Part model, mm, in its own coordinate system. A direction names the side the tool comes from. Coordinates: 2 decimals unless noted, no trailing zeros. Write each loop counter-clockwise with the first axis right and the second up, starting at its lowest first coordinate (ties: lowest second). Pieces come first, ordered by that corner, then holes. Notation, with made-up numbers: (-31.5, 42.5) -> (-22.5, 42.5) arc R18 ccw to (-22.5, 50.5) -> close; hole circle Ø10 at (75.25, 81). An arc over 180 degrees is marked (long way). Write item = value, one per line. Start each with the question number.
Q1. Pin check, flat tip, straight feed: P1, Ø1.5, axis at y = 365.5, z = -5, coming from the +X side. Stop position of the tip, or through.
Q2. Band-saw the part on B-B, the plane x = -12.7. Give the number of separate pieces and of enclosed holes in the cut face, plus the area to 3 significant figures.
Q3. Band-saw the part on C-C, the plane y = 209.55. List the corners of the cut face in (x, z).
Q4. Pull direction Z, two halves, no side cores. Call faces 3 (the cylindrical face through (-8.02, 16.99, -24.62)), 4 (the flat face through (-13, 219, 0)), 5 (the flat face through (-13, 219, -23.812)): released by +Z, released by -Z, zero draft, split by the parting line, or undercut.
Q5. Probe line 1 (Y direction, x = -12.7, z = -24.7); line 2 (X direction, y = 431.8, z = -24.35); line 3 (Z direction, x = -18.5, y = 244). List the from-to ranges inside material, lowest first.
Q6. Band-saw the part on A-A, the plane y = 12.7. List the corners of the cut face in (x, z).
Q7. Tool access for faces 1 (the flat face through (0, 219, -4)), 2 (the flat face through (-1.588, 219, -3)): list every direction of +Z, -Z, +X, -X, +Y, -Y with a clear straight run to the whole face (end or side of a thin tool).
Q8. Band-saw the part on D-D, the plane y = 105. List the corners of the cut face in (x, z), plus the area to 3 significant figures.
Autodesk Inventor part; units mm, degrees
ref_plane "YZ Plane" through (0, 0, 0) normal (1, 0, 0) x (0, 1, 0)
ref_plane "XZ Plane" through (0, 0, 0) normal (0, 1, 0) x (-1, 0, 0)
ref_plane "XY Plane" through (0, 0, 0) normal (0, 0, 1) x (1, 0, 0)
sketch "Sketch1" plane through (0, 0, 0) normal (0, 1, 0) x (-1, 0, 0)
  line L0 (0, 0) -> (25.4, 0)
  line L1 (25.4, 0) -> (25.4, -25.4)
  line L2 (25.4, -25.4) -> (0, -25.4)
  line L3 (0, -25.4) -> (0, 0)
  line L4 (23.8125, -23.8125) -> (23.8125, -1.5875)
  line L5 (23.8125, -1.5875) -> (1.5875, -1.5875)
  line L6 (1.5875, -1.5875) -> (1.5875, -23.8125)
  line L7 (1.5875, -23.8125) -> (23.8125, -23.8125)
  dimension "d0" = 25.4
  dimension "d1" = 25.4
  dimension "d2" = 1.5875
extrude "Extrusion1" add sketch "Sketch1" along normal blind 444.5
sketch "Sketch2" plane through (-25.4, 0, 0) normal (0, 0, 1) x (1, 0, 0)
  circle A0 centre (12.7, 431.8) radius 6.35
  line L0 (0, 444.5) -> (25.4, 444.5)
  point P0 (25.4, 0)
  dimension "d5" = 12.7
  dimension "d6" = 12.7
extrude "Extrusion2" cut sketch "Sketch2" against normal blind 25.4
sketch "Sketch4" plane through (0, 0, -25.4) normal (0, 0, -1) x (-1, 0, 0)
  circle A0 centre (12.7, 12.7) radius 6.35
  line L0 (25.4, 0) -> (0, 0)
  line L1 (0, 0) -> (0, 444.5)
  dimension "d17" = 12.7
  dimension "d18" = 12.7
  dimension "d19" = 12.7
extrude "Extrusion4" cut sketch "Sketch4" against normal blind 25.4
sketch "Sketch5" plane through (0, 0, -25.4) normal (0, 0, -1) x (-1, 0, 0)
  circle A0 centre (12.7, 209.55) radius 6.35
  line L0 (0, 0) -> (0, 444.5)
  line L1 (0, 444.5) -> (25.4, 444.5)
  dimension "d22" = 12.7
  dimension "d23" = 12.7
  dimension "d24" = 234.95
extrude "Extrusion5" cut sketch "Sketch5" against normal blind 25.4
sketch "Sketch6" plane through (0, 0, 0) normal (1, 0, 0) x (0, 0, -1)
  line L0 (5.08, 265.303) -> (20.32, 265.303)
  line L1 (20.32, 265.303) -> (20.32, 88.9)
  line L2 (20.32, 88.9) -> (5.08, 88.9)
  line L3 (5.08, 88.9) -> (5.08, 265.303)
  line L4 (23.8125, 444.5) -> (1.5875, 444.5)
  line L5 (25.4, 0) -> (25.4, 444.5)
  line L6 (0, 0) -> (0, 444.5)
  line L7 (25.4, 0) -> (0, 0)
  dimension "d28" = 5.08
  dimension "d29" = 5.08
  dimension "d30" = 176.403
  dimension "d33" = 88.9
extrude "Extrusion6" cut sketch "Sketch6" against normal blind 25.4
properties part number "AP 5"
Ans:
q1.P1 = 0
q2.separate_pieces = 8
q2.enclosed_holes = 0
q2.area = 1,290 mm2
q3.outline = (-25.4, -25.4) -> (-19.05, -25.4) -> (-19.05, -23.81) -> (-23.81, -23.81) -> (-23.81, -20.32) -> (-25.4, -20.32) -> close; (-25.4, -5.08) -> (-23.81, -5.08) -> (-23.81, -1.59) -> (-19.05, -1.59) -> (-19.05, 0) -> (-25.4, 0) -> close; (-6.35, -25.4) -> (0, -25.4) -> (0, -20.32) -> (-1.59, -20.32) -> (-1.59, -23.81) -> (-6.35, -23.81) -> close; (-6.35, -1.59) -> (-1.59, -1.59) -> (-1.59, -5.08) -> (0, -5.08) -> (0, 0) -> (-6.35, 0) -> close
q4.face_3 = zero draft
q4.face_4 = released by +Z
q4.face_5 = undercut
q5.line_1 = 0 to 6.35, 19.05 to 203.2, 215.9 to 425.45, 438.15 to 444.5
q5.line_2 = -25.4 to -19.05, -6.35 to 0
q5.line_3 = -25.4 to -23.81, -1.59 to 0
q6.outline = (-25.4, -25.4) -> (-19.05, -25.4) -> (-19.05, -23.81) -> (-23.81, -23.81) -> (-23.81, -1.59) -> (-19.05, -1.59) -> (-19.05, 0) -> (-25.4, 0) -> close; (-6.35, -25.4) -> (0, -25.4) -> (0, 0) -> (-6.35, 0) -> (-6.35, -1.59) -> (-1.59, -1.59) -> (-1.59, -23.81) -> (-6.35, -23.81) -> close
q7.face_1 = +Z, -Z, +X, +Y, -Y
q7.face_2 = +Y, -Y
q8.outline = (-25.4, -25.4) -> (0, -25.4) -> (0, -20.32) -> (-1.59, -20.32) -> (-1.59, -23.81) -> (-23.81, -23.81) -> (-23.81, -20.32) -> (-25.4, -20.32) -> close; (-25.4, -5.08) -> (-23.81, -5.08) -> (-23.81, -1.59) -> (-1.59, -1.59) -> (-1.59, -5.08) -> (0, -5.08) -> (0, 0) -> (-25.4, 0) -> close
q8.area = 103 mm2
